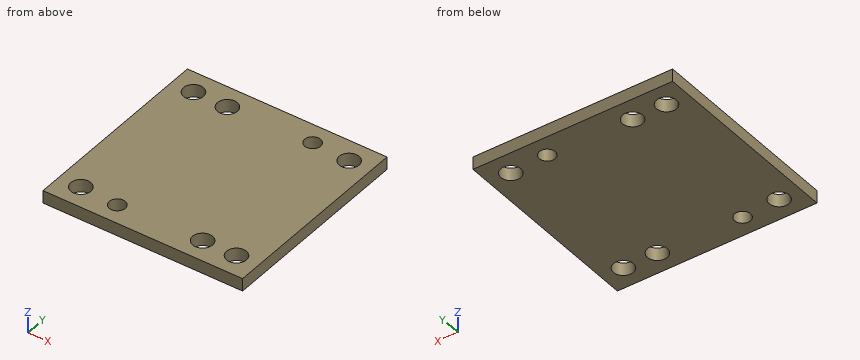
Autodesk Fusion 360 part; units mm, degrees
sketch "Esquisse1" plane through (0, 0, 0) normal (0, 0, 1) x (1, 0, 0)
  line L0 (0, 0) -> (50, 0)
  line L1 (50, 0) -> (50, 50)
  line L2 (50, 50) -> (0, 50)
  line L3 (0, 50) -> (0, 0)
  dimension "d1" = 50
  dimension "d2" = 50
extrude "Extrusion1" add sketch "Esquisse1" along normal blind 3.175
sketch "Esquisse2" plane through (0, 0, 3.175) normal (0, 0, 1) x (-1, 0, 0)
  line L0 (0, -50) -> (0, 0)
  line L1 (0, 0) -> (-50, 0)
  line L2 (-50, 0) -> (-50, -50)
  line L3 (-50, -50) -> (0, -50)
  line L4 (-50, -50) -> (0, 0) construction
  circle A0 centre (-5.5, -44.5) radius 2.5
  circle A1 centre (-44.5, -44.5) radius 2.5
  circle A2 centre (-44.5, -5.5) radius 2.5
  circle A3 centre (-5.5, -5.5) radius 2.5
  line L5 (-44.5, -5.5) -> (-5.5, -44.5) construction
  line L6 (-5.5, -5.5) -> (-44.5, -44.5) construction
  point P0 (-47, -5.5)
  point P1 (-44.5, -3)
  dimension "d5" = 3
  dimension "d6" = 3
  dimension "d7" = 5
extrude "Extrusion2" cut sketch "Esquisse2" against normal up to surface (3.175 mm away) contours A0 | A1 | A2 | A3
sketch "Esquisse3" plane through (0, 0, 3.175) normal (0, 0, 1) x (-1, 0, 0)
  circle A0 centre (-5.5, -5.5) radius 2.5
  circle A1 centre (-44.5, -5.5) radius 2.5
  circle A2 centre (-5.5, -44.5) radius 2.5
  circle A3 centre (-44.5, -44.5) radius 2.5
  line L0 (0, -50) -> (0, 0)
  line L1 (0, 0) -> (-50, 0)
  line L2 (-50, 0) -> (-50, -50)
  line L3 (-50, -50) -> (0, -50)
  line L4 (-50, -50) -> (0, 0) construction
  circle A4 centre (-35, -45) radius 2
  circle A5 centre (-15, -5) radius 2
  line L5 (-15, -5) -> (-35, -45) construction
  point P0 (-25, -25)
  point P1 (-35, -47)
  dimension "d10" = 4
  dimension "d11" = 10
  dimension "d12" = 3
extrude "Extrusion3" cut sketch "Esquisse3" against normal up to surface (3.175 mm away) contours A4 | A5
sketch "Esquisse4" plane through (0, 0, 3.175) normal (0, 0, 1) x (-1, 0, 0)
  circle A0 centre (-35, -45) radius 2
  circle A1 centre (-15, -5) radius 2
  circle A2 centre (-5.5, -5.5) radius 2.5
  circle A3 centre (-44.5, -5.5) radius 2.5
  circle A4 centre (-5.5, -44.5) radius 2.5
  circle A5 centre (-44.5, -44.5) radius 2.5
  line L0 (0, -50) -> (0, 0)
  line L1 (0, 0) -> (-50, 0)
  line L2 (-50, 0) -> (-50, -50)
  line L3 (-50, -50) -> (0, -50)
  line L4 (-10, -40) -> (-40, -40) construction
  line L5 (-40, -40) -> (-40, -10) construction
  line L6 (-40, -10) -> (-10, -10) construction
  line L7 (-10, -10) -> (-10, -40) construction
  line L8 (-10, -40) -> (-40, -10) construction
  line L9 (0, 0) -> (-50, -50) construction
  circle A6 centre (-14, -44.5) radius 2.5
  circle A7 centre (-36, -5.5) radius 2.5
  line L10 (-36, -5.5) -> (-14, -44.5) construction
  point P0 (-14, -42)
  dimension "d15" = 30
  dimension "d16" = 30
  dimension "d17" = 5
  dimension "d18" = 2
  dimension "d19" = 4
extrude "Extrusion4" cut sketch "Esquisse4" against normal up to surface (3.175 mm away) contours A6 | A7
sketch "Esquisse5" plane through (0, 0, 3.175) normal (0, 0, 1) x (-1, 0, 0)
  circle A0 centre (-14, -44.5) radius 2.5
  circle A1 centre (-36, -5.5) radius 2.5
  circle A2 centre (-35, -45) radius 2
  circle A3 centre (-15, -5) radius 2
  circle A4 centre (-5.5, -5.5) radius 2.5
  circle A5 centre (-44.5, -5.5) radius 2.5
  circle A6 centre (-5.5, -44.5) radius 2.5
  circle A7 centre (-44.5, -44.5) radius 2.5
  line L0 (0, -50) -> (0, 0)
  line L1 (0, 0) -> (-50, 0)
  line L2 (-50, 0) -> (-50, -50)
  line L3 (-50, -50) -> (0, -50)
  line L4 (-10, -40) -> (-40, -40)
  line L5 (-40, -40) -> (-40, -10)
  line L6 (-40, -10) -> (-10, -10)
  line L7 (-10, -10) -> (-10, -40)
  point P0 (-40, -25)
  point P1 (-50, -25)
  point P2 (-25, -40)
  point P3 (-25, -50)
  dimension "d22" = 30
sketch "Esquisse6" plane through (0, 0, 0) normal (0, 0, -1) x (1, 0, 0)
  circle A0 centre (14, -44.5) radius 2.5
  circle A1 centre (36, -5.5) radius 2.5
  circle A2 centre (35, -45) radius 2
  circle A3 centre (15, -5) radius 2
  circle A4 centre (5.5, -5.5) radius 2.5
  circle A5 centre (44.5, -5.5) radius 2.5
  circle A6 centre (5.5, -44.5) radius 2.5
  circle A7 centre (44.5, -44.5) radius 2.5
  line L0 (0, 0) -> (0, -50)
  line L1 (0, -50) -> (50, -50)
  line L2 (50, -50) -> (50, 0)
  line L3 (50, 0) -> (0, 0)
  line L4 (0, -10) -> (50, -10)
  line L5 (50, -10) -> (50, -40)
  line L6 (50, -40) -> (0, -40)
  line L7 (0, -40) -> (0, -10)
  point P0 (10, -40)
  point P1 (10, -10)
equation "d3 = 1 / 8 * 1 in"
Can you work these out from the model? Positions are in its coordinate system, mm. Coordinates: 2 decimals unless noted, no trailing zeros. Order: outer loops, then holes, each group sorted by start corner. A loop starts at its lowest first (then second) coordinate and runs counter-clockwise, first axis right, second up.
1. I need wall thicknesses on line 1 (X direction, y = 43.5, z = 2.85); line 2 (Y direction, x = 34, z = 0.85); line 3 (X direction, y = 6, z = 1.6). Which ranges of each line are inside material? Lowest first, please.
2. I'm going to push a flat-ended pin straight in: pin 1 (3.5 mm diameter, centred on x = 15, y = 5, fed in from +Z). Where does the tip first touch, or does it pass through?
3. If we section it at C-C (x = 36): Please give me the cut outline in (y, z) (3 decimals).
4. If we section it at A-A (z = 2.05): Give the number of separate pieces and of enclosed holes in the cut face, then the cut area to 3 significant figures.
5. If we section it at B-B (x = 44.5): Please give me the cut outline in (y, z) (3 decimals), then the cut area to 3 significant figures.
Entries:
1. line 1: x = 0 to 3.21, 7.79 to 11.71, 16.29 to 33.68, 36.32 to 42.21, 46.79 to 50
1. line 2: y = 0 to 4, 7 to 43.27, 46.73 to 50
1. line 3: x = 0 to 3.05, 7.95 to 13.27, 16.73 to 33.55, 38.45 to 42.05, 46.95 to 50
2. pin 1: passes through
3. outline: (0, 0) - (3, 0) - (3, 3.175) - (0, 3.175) - close; (8, 0) - (43.268, 0) - (43.268, 3.175) - (8, 3.175) - close; (46.732, 0) - (50, 0) - (50, 3.175) - (46.732, 3.175) - close
4. separate pieces: 1
4. enclosed holes: 8
4. area: 2,360 mm2
5. outline: (0, 0) - (3, 0) - (3, 3.175) - (0, 3.175) - close; (8, 0) - (42, 0) - (42, 3.175) - (8, 3.175) - close; (47, 0) - (50, 0) - (50, 3.175) - (47, 3.175) - close
5. area: 127 mm2
